Design review of the part built by this model. Coordinates are the model's own, in mm. A direction names the side the tool comes from. Give positions to 0.01 mm unless a question says otherwise; leave off trailing zeros. Write each loop counter-clockwise with the first axis right and the second up, starting at its lowest first coordinate (ties: lowest second). Pieces come first, ordered by that corner, then holes. Notation, with made-up numbers: (3, 20.5) -> (38, 20.5) arc R22 cw to (38, 42.5) -> close; hole circle Ø8 at (-40, -13.75). An arc over 180 degrees is marked (long way). Use CSV: the item, a comma, the result in double quotes.
```python
from build123d import *

# Parameters (mm, degrees)
BOSS_EXTRUDE1_DEPTH = 80
SKETCH2_R           = 7.5
CUT_EXTRUDE1_DEPTH  = 80


with BuildPart() as part:
    # Sketch1 → Boss-Extrude1 (new body)
    with BuildSketch(Plane.XY):
        Polygon((-10.10866575, -78.628610729), (-10.10866575, 61.371389271), (-20.10866575, 61.371389271), (-20.10866575, 36.371389271), (-23.10866575, 36.371389271), (-23.10866575, 33.371389271), (-20.10866575, 33.371389271), (-20.10866575, -16.628610729), (-23.10866575, -16.628610729), (-23.10866575, -19.628610729), (-20.10866575, -19.628610729), (-20.10866575, -69.628610729), (-23.10866575, -69.628610729), (-23.10866575, -72.628610729), (-20.10866575, -72.628610729), (-20.10866575, -78.628610729), align=None)
    extrude(amount=BOSS_EXTRUDE1_DEPTH)

    # Sketch2 → Cut-Extrude1 (cut)
    with BuildSketch(Plane.ZY.offset(20.10866575)):
        with Locations(Location((40, -48.628610729, 0), (0, 0, 270))):
            Circle(SKETCH2_R)
    extrude(amount=-CUT_EXTRUDE1_DEPTH, mode=Mode.SUBTRACT)


solid = part.part
```
(1) Take a section at B-B (x = -13). Write out the cut boundary in (y, z), then the cut area to 3 significant figures.
Established:
outline,"(-78.63, 0) -> (61.37, 0) -> (61.37, 80) -> (-78.63, 80) -> close; hole circle Ø15 at (-48.63, 40)"
area,"11,000 mm2"
(2) Clearance check with flat-ended pins moving along their axes: pin 1 (15 mm diameter, centred on y = 15, z = 42.5, fed in from -X); pin 2 (0.9 mm diameter, centred on x = -22.5, z = 40.5, fed in from +Y); pin 3 (0.9 mm diameter, centred on x = -22, z = 58, fed in from -Y). State where each tip first meets the part, or that it passes through.
Established:
pin 1,"stops at x = -20.11"
pin 2,"stops at y = 36.37"
pin 3,"stops at y = -72.63"
(3) For line 1 along Y through (x, z) = (-21.25, 22); line 2 along Z through (x, y) = (-11.5, -49); line 3 along X through (y, z) = (29.5, 10), list the stretches that pass through material, from the lowest coordinate up. Write a range as [from, to].
Established:
line 1,"y = [-72.63, -69.63], [-19.63, -16.63], [33.37, 36.37]"
line 2,"z = [0, 32.51], [47.49, 80]"
line 3,"x = [-20.11, -10.11]"
(4) Tool access review of faces 1 (the face through (-20.109, -76, 39)), 2 (the face through (-15, -78.629, 39)), 3 (the face through (-20.109, -39, 39)), 4 (the face through (-20.109, 49, 39)): name each direction out of +Z, -Z, +X, -X, +Y, -Y from which nothing blocks a thin tool from reaching the whole face with its end or side.
Established:
face 1,"+Z, -Z, -X, -Y"
face 2,"+Z, -Z, +X, -X, -Y"
face 3,"+Z, -Z, -X"
face 4,"+Z, -Z, -X, +Y"
(5) Take a section at D-D (y = -4). Write out the cut boundary in (x, z).
Established:
outline,"(-20.11, 0) -> (-10.11, 0) -> (-10.11, 80) -> (-20.11, 80) -> close"
(6) Take a section at C-C (z = 50.5). Write out the cut boundary in (x, y), then the cut area to 3 significant figures.
Established:
outline,"(-23.11, -72.63) -> (-20.11, -72.63) -> (-20.11, -78.63) -> (-10.11, -78.63) -> (-10.11, 61.37) -> (-20.11, 61.37) -> (-20.11, 36.37) -> (-23.11, 36.37) -> (-23.11, 33.37) -> (-20.11, 33.37) -> (-20.11, -16.63) -> (-23.11, -16.63) -> (-23.11, -19.63) -> (-20.11, -19.63) -> (-20.11, -69.63) -> (-23.11, -69.63) -> close"
area,"1,430 mm2"
(7) Take a section at A-A (z = 40). Write out the cut boundary in (x, y), then the cut area to 3 significant figures.
Established:
outline,"(-23.11, -72.63) -> (-20.11, -72.63) -> (-20.11, -78.63) -> (-10.11, -78.63) -> (-10.11, -56.13) -> (-20.11, -56.13) -> (-20.11, -69.63) -> (-23.11, -69.63) -> close; (-23.11, -19.63) -> (-20.11, -19.63) -> (-20.11, -41.13) -> (-10.11, -41.13) -> (-10.11, 61.37) -> (-20.11, 61.37) -> (-20.11, 36.37) -> (-23.11, 36.37) -> (-23.11, 33.37) -> (-20.11, 33.37) -> (-20.11, -16.63) -> (-23.11, -16.63) -> close"
area,"1,280 mm2"
(8) Mouldability with a two-part tool opening along Y and no side actions: class faces 5 (the face through (-20.109, 9, 39)), 6 (the face through (-22, -72.629, 39)), 7 (the face through (-15, 61.371, 39)) as +Y half, -Y half, draft (parallel to the pull), parting line (faces both ways), or undercut.
Established:
face 5,"undercut"
face 6,"-Y half"
face 7,"+Y half"
